Source: CAD feature listing. Evaluate the final solid. Frame: model axes, mm. A direction names the side the tool comes from. Give positions to 0.01 mm unless a question says otherwise; leave off trailing zeros. Loops run counter-clockwise (first coordinate to the right, second up) from the corner with the lowest first, then second, coordinate; pieces in that order, holes last. Notation, with made-up numbers: M 23.25,14.5 L 53.25,14.5 A19 ccw 53.25,46.5 Z; hole C -0.75,77 d11. An arc over 180 degrees is marked long. Answer in a Markdown table with one row per item.
```python
from build123d import *

# Parameters (mm, degrees)
F0_W      = 101.6
F0_H      = 101.6
F1_DEPTH  = 50.8
F2_W      = 25.4
F2_H      = 50.8
F3_DEPTH  = 50.8
F4_W      = 25.4
F4_H      = 50.8
F5_DEPTH  = 50.8
F7_DEPTH  = 25.4
F8_DEPTH  = 25.4
F10_DEPTH = 25.4
F11_R     = 12.7
F12_DEPTH = 50.8
F14_DEPTH = 50.8
F15_R     = 25.4
F16_R     = 25.4


with BuildPart() as f1:
    # F0 (on Top) → F1 (new body)
    with BuildSketch(Plane.XY):
        with Locations((-39.0884162307, 27.9844595671)):
            Rectangle(F0_W, F0_H)
    extrude(amount=F1_DEPTH)

    # F2 (on face) → F3 (join)
    with BuildSketch(Plane.YZ.offset(11.7115837693)):
        with Locations((66.0844595671, 25.4)):
            Rectangle(F2_W, F2_H)
    extrude(amount=F3_DEPTH)

    # F4 (on face) → F5 (join)
    with BuildSketch(Plane(origin=(-89.8884162307, 0, 0), x_dir=(0, -1, 0), z_dir=(-1, 0, 0))):
        with Locations((-66.0844595671, 25.4)):
            Rectangle(F4_W, F4_H)
    extrude(amount=F5_DEPTH)

    # F6 (on face) → F7 (join)
    with BuildSketch(Plane.XY.offset(50.8)):
        Polygon((-140.6884162307, 53.3844595671), (-89.8884162307, 53.3844595671), (11.7115837693, 53.3844595671), (62.5115837693, 53.3844595671), (62.5115837693, 78.7844595671), (-140.6884162307, 78.7844595671), align=None)
    extrude(amount=F7_DEPTH)

    # F8 (add): a face of the model
    f8_faces = [f1.faces().sort_by_distance(p)[0] for p in [
        (-39.0884162307, 66.0844595671, 76.2),
    ]]
    extrude(f8_faces, amount=F8_DEPTH)

    # F9 (on face) → F10 (join)
    with BuildSketch(Plane.XZ.offset(-53.3844595671)):
        Polygon((-140.6884162307, 50.8), (-89.8884162307, 50.8), (11.7115837693, 50.8), (62.5115837693, 50.8), (62.5115837693, 101.6), (-140.6884162307, 101.6), align=None)
    extrude(amount=F10_DEPTH)

    # F11 (on face) → F12 (cut)
    with BuildSketch(Plane.XZ.offset(-27.9844595671)):
        with Locations((-121.0152357817, 75.7217407227)):
            Circle(F11_R)
    extrude(amount=-F12_DEPTH, mode=Mode.SUBTRACT)

    # F13 (on face) → F14 (cut)
    with BuildSketch(Plane.XZ.offset(-27.9844595671)):
        with BuildLine():
            ThreePointArc((55.5737721028, 77.0839367255), (30.1813854063, 77.523618368), (55.5433280167, 76.2051005946))
            ThreePointArc((55.5433280167, 76.2051005946), (55.5661587993, 76.6442550829), (55.5737721028, 77.0839367255))
        make_face()
    extrude(amount=-F14_DEPTH, mode=Mode.SUBTRACT)

    # F15
    f15_edges = [f1.edges().sort_by_distance(p)[0] for p in [
        (62.511584, 53.38446, 101.6),
    ]]
    fillet(f15_edges, radius=F15_R)

    # F16
    f16_edges = [f1.edges().sort_by_distance(p)[0] for p in [
        (-140.688416, 53.38446, 101.6),
    ]]
    fillet(f16_edges, radius=F16_R)


solid = f1.part
```
1) Section B-B, the plane x = -82. Return loops of the section in (y, z), then the cut area to 3 significant figures.
Reply:
| item | result |
|---|---|
| outline | M -22.82,0 L 78.78,0 L 78.78,101.6 L 27.98,101.6 L 27.98,50.8 L -22.82,50.8 Z |
| area | 7,740 mm² |
2) Set-up query: faces 1 (the flat face through (-116, 53.384, 25)), 2 (the flat face through (-41, 27.984, 77)), 3 (the flat face through (-38, 54, 101.6)), 4 (the flat face through (11.712, 15, 25)). Return all of +Z, -Z, +X, -X, +Y, -Y with unobstructed straight access to the full face (end or side cutting, diameter ignored); none if empty.
Reply:
| item | result |
|---|---|
| face 1 | -Z, -X, -Y |
| face 2 | +Z, +X, -X, -Y |
| face 3 | +Z, +X, -X, +Y, -Y |
| face 4 | -Z, +X, -Y |
3) Section D-D, the plane z = 39. Return loops of the section in (x, y), then the cut area to 3 significant figures.
Reply:
| item | result |
|---|---|
| outline | M -140.69,53.38 L -89.89,53.38 L -89.89,-22.82 L 11.71,-22.82 L 11.71,53.38 L 62.51,53.38 L 62.51,78.78 L -140.69,78.78 Z |
| area | 12,900 mm² |
4) Section C-C, the plane z = 82.5. Return loops of the section in (x, y), then the cut area to 3 significant figures.
Reply:
| item | result |
|---|---|
| outline | M -139.89,27.98 L -131.76,27.98 L -131.76,78.78 L -139.89,78.78 Z; M -110.28,27.98 L 31.39,27.98 L 31.39,78.78 L -110.28,78.78 Z; M 54.36,27.98 L 61.72,27.98 L 61.72,78.78 L 54.36,78.78 Z |
| area | 7,980 mm² |
5) Material intervals for L1, parallel to X at y = 72, z = 86.5; L2, parallel to Z at x = 5, y = -18; L3, parallel to Y at x = -81.5, z = 73, sorted ascending.
Reply:
| item | result |
|---|---|
| L1 | x = -138.51 to -127.73, -114.3 to 34.35, 51.4 to 60.33 |
| L2 | z = 0 to 50.8 |
| L3 | y = 27.98 to 78.78 |
6) Pull-direction query (X, two-part tool) for faces 5 (the flat face through (37, 41, 50.8)), 6 (the cylindrical face through (-133.703, 53.029, 76.28)), 7 (the flat face through (62.512, 59, 46)), 8 (the flat face through (-140.688, 59, 47)); classes: released by +X, released by -X, zero draft, split by the parting line, or undercut.
Reply:
| item | result |
|---|---|
| face 5 | zero draft |
| face 6 | undercut |
| face 7 | released by +X |
| face 8 | released by -X |
7) Pin query (flat end, axial travel): pin 1 Ø20.5 at (x, y) = (43, 36.5) entering from -Z; pin 2 Ø5 at (x, z) = (14.5, 29.5) entering from -Y; pin 3 Ø3 at (x, y) = (-68.5, 21.5) entering from +Z. Return the tip coordinate at first contact, or that it passes through.
Reply:
| item | result |
|---|---|
| pin 1 | stops at z = 50.8 |
| pin 2 | stops at y = 53.38 |
| pin 3 | stops at z = 50.8 |
8) Section A-A, the plane y = 36.5. Return loops of the section in (x, z), then the cut area to 3 significant figures.
Reply:
| item | result |
|---|---|
| outline | M -140.69,50.8 L -89.89,50.8 L -89.89,0 L 11.71,0 L 11.71,50.8 L 62.51,50.8 L 62.51,76.2 A25.4 ccw 37.11,101.6 L -115.29,101.6 A25.4 ccw -140.69,76.2 Z; hole C -121.02,75.72 d25.4; hole C 42.87,77.08 d25.4 |
| area | 14,200 mm² |
